Input: part model. Units: mm. Frame: model coordinates. Face numbers are marked on the shaded views. A direction names the side the tool comes from. Coordinates: 2 decimals unless noted, no trailing zeros. Answer as a JSON object with one key per item and string values.
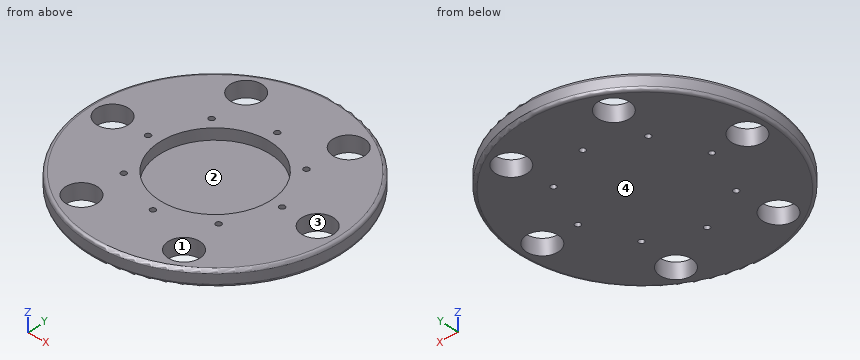
from build123d import *

# Parameters (mm, degrees)
SKETCH_3_R          = 80
EXTRUDE_1_DEPTH     = 10
SKETCH_4_R          = 35
CUT_EXTRUDE_1_DEPTH = 7
SKETCH_5_R          = 10
CUT_EXTRUDE_2_DEPTH = 10
SKETCH_6_R          = 1.75
CUT_EXTRUDE_3_DEPTH = 10
FILLET_1_R          = 2


with BuildPart() as part:
    # 草图3 → 凸台-拉伸1 (new body)
    with BuildSketch(Plane.XY):
        Circle(SKETCH_3_R)
    extrude(amount=-EXTRUDE_1_DEPTH)

    # 草图4 → 切除-拉伸1 (cut)
    with BuildSketch(Plane.XY):
        Circle(SKETCH_4_R)
    extrude(amount=-CUT_EXTRUDE_1_DEPTH, mode=Mode.SUBTRACT)

    # 草图5 → 切除-拉伸2 (cut)
    with BuildSketch(Plane.XY):
        with Locations((-65, 0)):
            Circle(SKETCH_5_R)
        with Locations((-32.4995, 56.292517271)):
            Circle(SKETCH_5_R)
        with Locations((32.5015, 56.292517271)):
            Circle(SKETCH_5_R)
        with Locations((65.002, 0)):
            Circle(SKETCH_5_R)
        with Locations((32.5015, -56.292517271)):
            Circle(SKETCH_5_R)
        with Locations((-32.4995, -56.292517271)):
            Circle(SKETCH_5_R)
    extrude(amount=-CUT_EXTRUDE_2_DEPTH, mode=Mode.SUBTRACT)

    # 草图6 → 切除-拉伸3 (cut)
    with BuildSketch(Plane.XY):
        with Locations((-42.5, 0)):
            Circle(SKETCH_6_R)
        with Locations((-30.0520382, 30.0520382)):
            Circle(SKETCH_6_R)
        with Locations((0, 42.5)):
            Circle(SKETCH_6_R)
        with Locations((30.0520382, 30.0520382)):
            Circle(SKETCH_6_R)
        with Locations((42.5, 0)):
            Circle(SKETCH_6_R)
        with Locations((30.0520382, -30.0520382)):
            Circle(SKETCH_6_R)
        with Locations((0, -42.5)):
            Circle(SKETCH_6_R)
        with Locations((-30.0520382, -30.0520382)):
            Circle(SKETCH_6_R)
    extrude(amount=-CUT_EXTRUDE_3_DEPTH, mode=Mode.SUBTRACT)

    # 圆角1
    fillet_1_edges = [part.edges().sort_by_distance(p)[0] for p in [
        (-80, 0, 0),
        (-80, 0, -10),
    ]]
    fillet(fillet_1_edges, radius=FILLET_1_R)


solid = part.part
1. Pin query (flat end, axial travel): P1, Ø3, axis at x = -37, z = -2, coming from the +Y side; P2, Ø3, axis at x = 30.05, y = 30.05, coming from the -Z side; P3, Ø5, axis at x = -45, z = -1, coming from the +Y side; P4, Ø2, axis at x = 51.5, z = -4.5, coming from the -Y side. Return the tip coordinate at first contact, or that it passes through.
Reply:
{"P1": "stops at y = 71.69", "P2": "passes through", "P3": "stops at y = 67.69", "P4": "stops at y = -62.05"}
2. Access query for the marked faces 1 and 2. Directions: +Z, -Z, +X, -X, +Y, -Y. A direction counts if a zero-diameter tool reaches every point of the face in a straight line with its end or side. Return the directions, or none.
Reply:
{"face 1": "+Z, -Z", "face 2": "+Z"}
3. Mould query, pull axis X, two halves, no side actions, for the marked faces 3 and 4. Classes: pulls with the +X half, pulls with the -X half, needs draft (parallel to the pull), parting line crosses it, or undercut.
Reply:
{"face 3": "undercut", "face 4": "needs draft"}
4. Line query: line 1 along Y through (x, z) = (0, -3.75); line 2 along Y through (x, z) = (-30.5, -8); line 3 along X through (y, z) = (3, -8). Output: solid intervals per line, ascending.
Reply:
{"line 1": "y = -80 to -44.25, -40.75 to -35, 35 to 40.75, 44.25 to 80", "line 2": "y = -73.96 to -66.09, -46.49 to -31.74, -28.36 to 28.36, 31.74 to 46.49, 66.09 to 73.96", "line 3": "x = -79.94 to -74.54, -55.46 to 55.46, 74.54 to 79.94"}
5. Section query A-A (z = -5.5). Count the separate pieces of the cut face and the enclosed holes in it, plus the area to 3 significant figures.
Reply:
{"separate pieces": "1", "enclosed holes": "15", "area": "14,300 mm2"}
